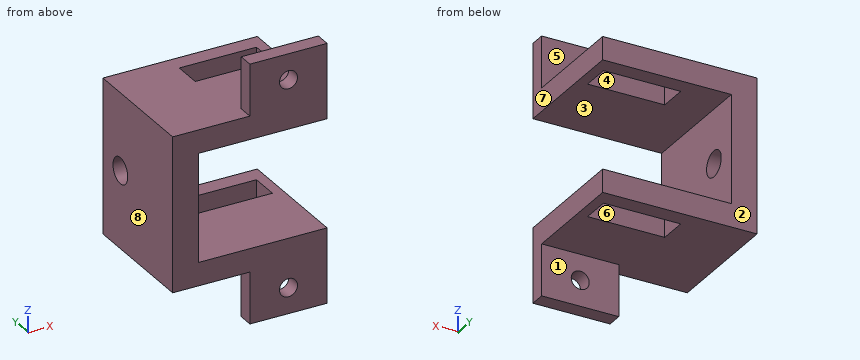
from build123d import *

# Parameters (mm, degrees)
SKETCH1_W           = 30
SKETCH1_H           = 24
SKETCH1_W_2         = 15
SKETCH1_H_2         = 5.5
BOSS_EXTRUDE1_DEPTH = 30
SKETCH2_W           = 21
SKETCH2_H           = 24
CUT_EXTRUDE1_DEPTH  = 25
SKETCH3_R           = 2.525
CUT_EXTRUDE2_DEPTH  = 41.853396432
SKETCH_1_W          = 15
SKETCH_1_H          = 3
EXTRUDE_1_DEPTH     = 10
SKETCH_2_W          = 15
SKETCH_2_H          = 3
EXTRUDE_2_DEPTH     = 10
SKETCH_3_R          = 1.75
CUT_EXTRUDE_1_DEPTH = 48.602520942
SKETCH_4_R          = 1.75
CUT_EXTRUDE_2_DEPTH = 48.602520942


with BuildPart() as part:
    # Sketch1 → Boss-Extrude1 (new body)
    with BuildSketch(Plane.XY):
        Rectangle(SKETCH1_W, SKETCH1_H)
        with Locations((5.5, 6)):
            Rectangle(SKETCH1_W_2, SKETCH1_H_2, mode=Mode.SUBTRACT)
    extrude(amount=BOSS_EXTRUDE1_DEPTH)

    # Sketch2 → Cut-Extrude1 (cut)
    with BuildSketch(Plane(origin=(15, 0, 0), x_dir=(0, 0, -1), z_dir=(1, 0, 0))):
        with Locations((-15, 0)):
            Rectangle(SKETCH2_W, SKETCH2_H)
    extrude(amount=-CUT_EXTRUDE1_DEPTH, mode=Mode.SUBTRACT)

    # Sketch3 → Cut-Extrude2 (cut, through all)
    with BuildSketch(Plane(origin=(-10, 0, 0), x_dir=(0, 0, -1), z_dir=(1, 0, 0))):
        with Locations((-15, 6)):
            Circle(SKETCH3_R)
    extrude(amount=-CUT_EXTRUDE2_DEPTH, mode=Mode.SUBTRACT)

    # Эскиз1 → Бобышка-Вытянуть1 (add)
    with BuildSketch(Plane.XY.offset(30)):
        with Locations((7.5, -10.5)):
            Rectangle(SKETCH_1_W, SKETCH_1_H)
    extrude(amount=EXTRUDE_1_DEPTH)

    # Эскиз2 → Бобышка-Вытянуть2 (add)
    with BuildSketch(Plane(origin=(0, 0, 0), x_dir=(-1, 0, 0), z_dir=(0, 0, -1))):
        with Locations((-7.5, -10.5)):
            Rectangle(SKETCH_2_W, SKETCH_2_H)
    extrude(amount=EXTRUDE_2_DEPTH)

    # Эскиз3 → Вырез-Вытянуть1 (cut, through all)
    with BuildSketch(Plane(origin=(0, -9, 0), x_dir=(1, 0, 0), z_dir=(0, 1, 0))):
        with Locations(Location((7.5, -35, 0), (0, 0, 270))):
            Circle(SKETCH_3_R)
    extrude(amount=-CUT_EXTRUDE_1_DEPTH, mode=Mode.SUBTRACT)

    # Эскиз4 → Вырез-Вытянуть2 (cut, through all)
    with BuildSketch(Plane(origin=(0, -9, 0), x_dir=(1, 0, 0), z_dir=(0, 1, 0))):
        with Locations(Location((7.5, 5, 0), (0, 0, 270))):
            Circle(SKETCH_4_R)
    extrude(amount=-CUT_EXTRUDE_2_DEPTH, mode=Mode.SUBTRACT)


solid = part.part
Build history of the part. All positions in model axes, mm. Face numbers are marked on the shaded views. A direction names the side the tool comes from. Give positions to 0.01 mm unless a question says otherwise; leave off trailing zeros. Loops run counter-clockwise (first coordinate to the right, second up) from the corner with the lowest first, then second, coordinate; pieces in that order, holes last. Notation, with made-up numbers: (62.5, 32) - (106.5, 32) arc R12 ccw to (106.5, 54) - close; hole circle Ø9 at (15.25, 14.25). An arc over 180 degrees is marked (long way). Write item = value, one per line. Start each with the question number.
1) Tool access for the marked faces 1, 2, 3, 4 and 5: list every direction of +Z, -Z, +X, -X, +Y, -Y with a clear straight run to the whole face (end or side of a thin tool).
2) Band-saw the part on C-C on z = 15. Give the cut face in (x, y) (3 decimals).
3) Band-saw the part on D-D on x = 7.5. Give the cut face in (y, z), plus the area to 4 significant figures.
4) Probe probe 1 along Y at (x, z) = (6, 26); probe 2 along Z at (x, y) = (7, 0.5); probe 3 along X at (y, z) = (-10.15, -5). List the from-to ranges inside material, lowest first. Write a range as from..to.
5) Drop flat-ended pins along their axis: pin 1 Ø1.5 at (y, z) = (-11, 33.5) entering from -X; pin 2 Ø6 at (x, y) = (8, 3) entering from +Z; pin 3 Ø3 at (x, z) = (10.5, 33.5) entering from +Y. Give the stop position or say it passes through.
6) Band-saw the part on B-B on x = -6.75. Give the cut face in (y, z), plus the area to 3 significant figures.
7) Band-saw the part on A-A on y = 6. Give the cut face in (x, z) (3 decimals).
8) Pull direction X, two halves, no side cores. Call the marked faces 6, 7 and 8: +X half, -X half, draft (parallel to the pull), parting line (faces both ways), or undercut.
Final values:
q1.face_1 = -Z, +X, -X, +Y
q1.face_2 = +Z, -Z, +X, -X, +Y
q1.face_3 = +X, +Y, -Y
q1.face_4 = +Z, -Z
q1.face_5 = +Z, +X, -X, +Y
q2.outline = (-15, -12) - (-10, -12) - (-10, 3.475) - (-15, 3.475) - close; (-15, 8.525) - (-10, 8.525) - (-10, 12) - (-15, 12) - close
q3.outline = (-12, -10) - (-9, -10) - (-9, -6.75) - (-12, -6.75) - close; (-12, -3.25) - (-9, -3.25) - (-9, 0) - (3.25, 0) - (3.25, 4.5) - (-12, 4.5) - close; (-12, 25.5) - (3.25, 25.5) - (3.25, 30) - (-9, 30) - (-9, 33.25) - (-12, 33.25) - close; (-12, 36.75) - (-9, 36.75) - (-9, 40) - (-12, 40) - close; (8.75, 0) - (12, 0) - (12, 4.5) - (8.75, 4.5) - close; (8.75, 25.5) - (12, 25.5) - (12, 30) - (8.75, 30) - close
q3.area = 205.5 mm²
q4.probe_1 = -12..3.25, 8.75..12
q4.probe_2 = 0..4.5, 25.5..30
q4.probe_3 = 0..5.75, 9.25..15
q5.pin_1 = 0
q5.pin_2 = 30
q5.pin_3 = -9
q6.outline = (-12, 0) - (12, 0) - (12, 4.5) - (-12, 4.5) - close; (-12, 25.5) - (12, 25.5) - (12, 30) - (-12, 30) - close
q6.area = 216 mm²
q7.outline = (-15, 0) - (-2, 0) - (-2, 4.5) - (-10, 4.5) - (-10, 12.475) - (-15, 12.475) - close; (-15, 17.525) - (-10, 17.525) - (-10, 25.5) - (-2, 25.5) - (-2, 30) - (-15, 30) - close; (13, 0) - (15, 0) - (15, 4.5) - (13, 4.5) - close; (13, 25.5) - (15, 25.5) - (15, 30) - (13, 30) - close
q8.face_6 = undercut
q8.face_7 = +X half
q8.face_8 = -X half
